Here's the drawing with two shaded views (mm, measured from the low corner). I have some questions. Round coordinates to 2 decimals unless told otherwise and drop trailing zeros. Loops run counter-clockwise (first coordinate to the right, second up) from the corner with the lowest first, then second, coordinate; pieces in that order, holes last.
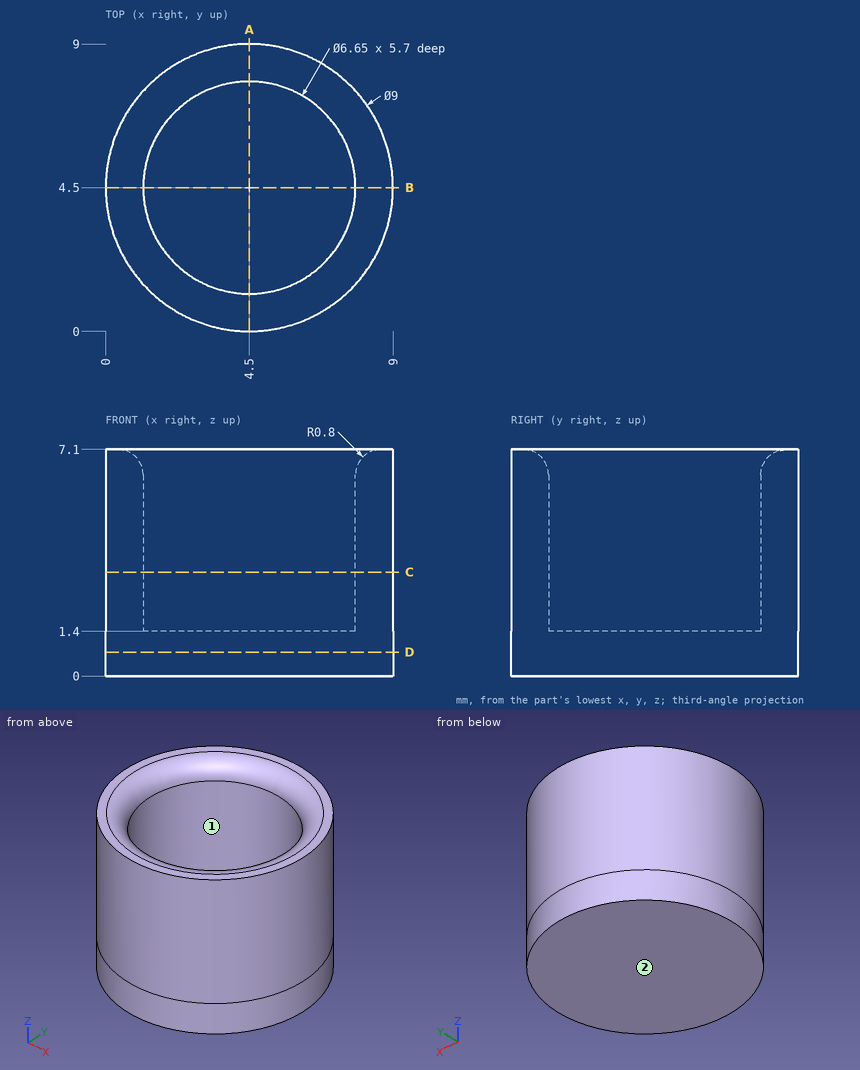
(1) Will these pins go through, and if not, where does the flat tip stop? P1, Ø4, axis at x = 2, z = 4.5, coming from the +Y side; P2, Ø1, axis at x = 1.5, z = 4.5, coming from the -Y side; P3, Ø1.5, axis at x = 7, z = 1, coming from the +Y side.
Worked answers:
P1: stops at y = 8.97
P2: stops at y = 0.76
P3: stops at y = 8.65
(2) If I drill on line 1 (Y direction, x = 4.5, z = 4.75) (3 decimals); line 2 (Z direction, x = 2.5, y = 4.5); line 3 (X direction, y = 4, z = 4.25), over which ranges is the centre line in solid material (lowest first)?
Worked answers:
line 1: y = 0 to 1.175, 7.825 to 9
line 2: z = 0 to 1.4
line 3: x = 0.03 to 1.21, 7.79 to 8.97
(3) If we mould it in two halves opening along X, with no side actions, what happens to the marked faces 1 and 2? For each: released by +X, released by -X, zero draft, split by the parting line, or undercut.
Worked answers:
face 1: undercut
face 2: zero draft
(4) If we section it at D-D, the plane z = 0.75: List the corners of the cut face in (x, y) for me.
Worked answers:
outline: circle Ø9 at (4.5, 4.5)
(5) If we section it at C-C, the plane z = 3.25: List the corners of the cut face in (x, y) for me (3 decimals).
Worked answers:
outline: circle Ø9 at (4.5, 4.5); hole circle Ø6.65 at (4.5, 4.5)
(6) If we section it at A-A, the plane x = 4.5: List the corners of the cut face in (y, z) for me (3 decimals).
Worked answers:
outline: (0, 0) - (9, 0) - (9, 7.1) - (8.625, 7.1) arc R0.8 ccw to (7.825, 6.3) - (7.825, 1.4) - (1.175, 1.4) - (1.175, 6.3) arc R0.8 ccw to (0.375, 7.1) - (0, 7.1) - close
